Source: three-view drawing plus pictorial views. Frame: mm from the lowest corner of the part. A direction names the side the tool comes from. Give positions to 0.01 mm unless a question says otherwise; leave off trailing zeros. Order: outer loops, then holes, each group sorted by start corner. A loop starts at its lowest first (then second) coordinate and runs counter-clockwise, first axis right, second up. Notation, with made-up numbers: (-37, 75.5) -> (-3, 75.5) arc R5 cw to (-3, 84.5) -> close; hole circle Ø5 at (68.5, -3). An arc over 180 degrees is marked (long way). Answer in a Markdown table with one row per item. Add a question column.
Q1. Set-up query: the marked faces 1 and 2. Return all of +Z, -Z, +X, -X, +Y, -Y with unobstructed straight access to the full face (end or side cutting, diameter ignored); none if empty.
Q2. Cut plane A-A on x = 5. Return the cut outline in (y, z), and give its area (3 significant figures).
Q3. Contact query for flat-ended pins moving along their axis: P1, Ø3, axis at x = 19, z = 2, coming from the -Y side; P2, Ø6, axis at x = 12, y = 17.5, coming from the -Z side; P3, Ø5, axis at x = 29.5, y = 12, coming from the -Z side. Output: stop coordinate, or through.
Q4. Cut plane C-C on z = 7.5. Return the cut outline in (x, y).
Q5. Cut plane D-D on x = 17.5. Return the cut outline in (y, z), and give its area (3 significant figures).
Q6. Cut plane B-B on y = 12.5. Return the cut outline in (x, z).
Q7. Line query: line 1 along Y through (x, z) = (5, 6.3); line 2 along Z through (x, y) = (2, 13.5); line 3 along Y through (x, z) = (17.5, 3.5). Output: solid intervals per line, ascending. Write a range as from..to.
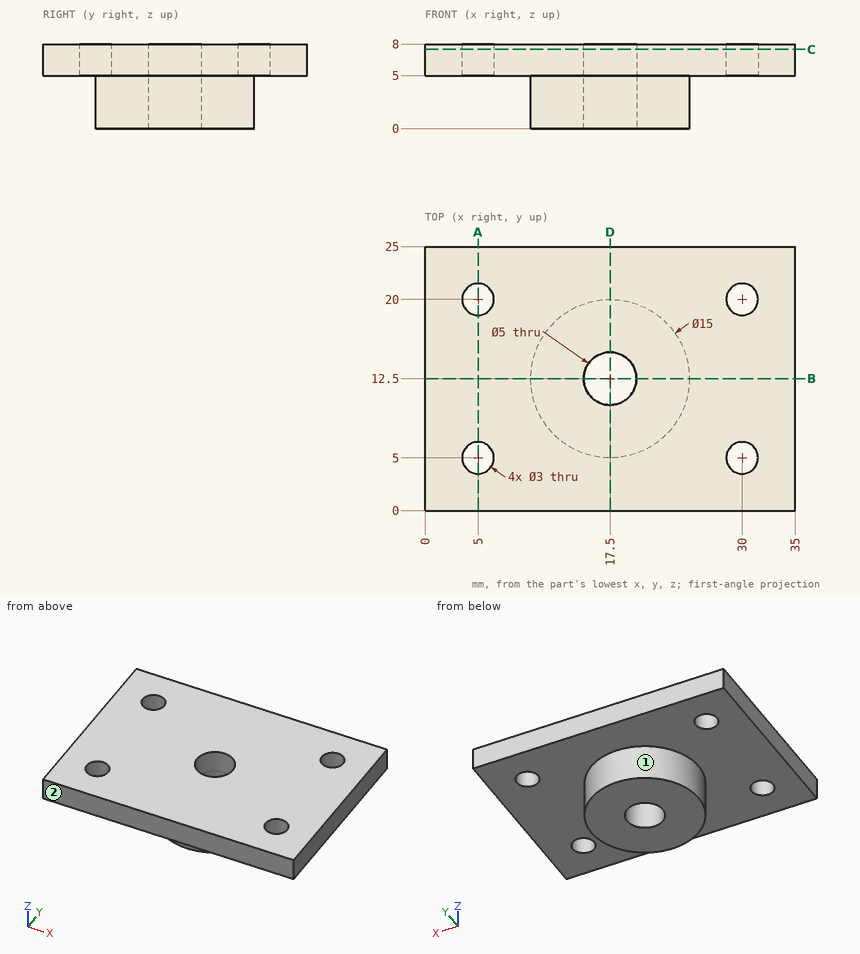
Completed:
| question | item | result |
|---|---|---|
| 1 | face 1 | -Z |
| 1 | face 2 | +Z, -Z, +X, -X, -Y |
| 2 | outline | (0, 5) -> (3.5, 5) -> (3.5, 8) -> (0, 8) -> close; (6.5, 5) -> (18.5, 5) -> (18.5, 8) -> (6.5, 8) -> close; (21.5, 5) -> (25, 5) -> (25, 8) -> (21.5, 8) -> close |
| 2 | area | 57.0 mm² |
| 3 | P1 | stops at y = 5 |
| 3 | P2 | stops at z = 0 |
| 3 | P3 | stops at z = 5 |
| 4 | outline | (0, 0) -> (35, 0) -> (35, 25) -> (0, 25) -> close; hole circle Ø3 at (5, 5); hole circle Ø3 at (5, 20); hole circle Ø5 at (17.5, 12.5); hole circle Ø3 at (30, 5); hole circle Ø3 at (30, 20) |
| 5 | outline | (0, 5) -> (5, 5) -> (5, 0) -> (10, 0) -> (10, 8) -> (0, 8) -> close; (15, 0) -> (20, 0) -> (20, 5) -> (25, 5) -> (25, 8) -> (15, 8) -> close |
| 5 | area | 110 mm² |
| 6 | outline | (0, 5) -> (10, 5) -> (10, 0) -> (15, 0) -> (15, 8) -> (0, 8) -> close; (20, 0) -> (25, 0) -> (25, 5) -> (35, 5) -> (35, 8) -> (20, 8) -> close |
| 7 | line 1 | y = 0..3.5, 6.5..18.5, 21.5..25 |
| 7 | line 2 | z = 5..8 |
| 7 | line 3 | y = 5..10, 15..20 |
